Model file for the job. Use its own axes, mm. A direction names the side the tool comes from. Give positions to 0.01 mm unless a question says otherwise; leave off trailing zeros. Write each loop counter-clockwise with the first axis right and the second up, starting at its lowest first coordinate (ties: lowest second). Pieces come first, ordered by that corner, then holes. Notation, with made-up numbers: (17, 76) - (63, 76) arc R11 ccw to (63, 88) - close; hole circle Ø2 at (19.25, 54). An arc over 180 degrees is marked (long way). One line per item, written item: value. Start each with the question number.
(1) Drop flat-ended pins along their axis: P1, Ø2, axis at x = -17, z = -2, coming from the +Y side; P2, Ø2.5, axis at y = 32.5, z = 0, coming from the +X side. Give the stop position or say it passes through.
(2) Probe L1, parallel to Y at x = -18.8, z = 0; L2, parallel to X at y = 51, z = 4.25 (3 decimals); L3, parallel to Z at x = -18.45, y = 32. List the from-to ranges inside material, lowest first.
(3) Cut at D-D, the plane z = -0.25. State how many separate pieces and enclosed holes the cut face has, and give its area (3 significant figures).
(4) Cut at C-C, the plane y = 42.5. List the corners of the cut face in (x, z) (3 decimals).
(5) Cut at B-B, the plane x = -18.55. List the corners of the cut face in (y, z).
(6) Cut at A-A, the plane y = 32.5. List the corners of the cut face in (x, z) (3 decimals), and give its area (3 significant figures).
(7) 3-axis set-ups, long thin cutter, end or side, ignore diameter. For faces 1 (the face through (-17, 36, 0)), 2 (the face through (-19, 40, -5)), 3 (the face through (-17, 44, 0)): which of +Z, -Z, +X, -X, +Y, -Y reach the whole face in a straight line?
(8) Mould opens along Z. For faces 4 (the face through (-19, 40, 5)), 5 (the face through (-14.646, 40.042, 0.089)), 6 (the face through (-19, 27.5, 0)), 7 (the face through (-19, 31, 0)) say: pulls with the +Z half, pulls with the -Z half, needs draft (parallel to the pull), parting line crosses it, or undercut.
from build123d import *

# Parameters (mm, degrees)
SKETCH1_W           = 10
SKETCH1_H           = 25
SKETCH1_R           = 1.5
BOSS_EXTRUDE1_DEPTH = 2
BOSS_EXTRUDE2_START = -56
BOSS_EXTRUDE2_DEPTH = 8
FILLET1_R           = 1


with BuildPart() as part:
    # Sketch1 → Boss-Extrude1 (new body)
    with BuildSketch(Plane(origin=(-20.145, 0, 0), x_dir=(0, 0, -1), z_dir=(1, 0, 0))):
        with Locations((0, 40)):
            Rectangle(SKETCH1_W, SKETCH1_H)
        with Locations((0, 47.5)):
            Circle(SKETCH1_R, mode=Mode.SUBTRACT)
        with Locations((0, 32.5)):
            Circle(SKETCH1_R, mode=Mode.SUBTRACT)
    extrude(amount=BOSS_EXTRUDE1_DEPTH)

    # Sketch2 → Boss-Extrude2 (add)
    with BuildSketch(Plane(origin=(0, 100, 0), x_dir=(1, 0, 0), z_dir=(0, 1, 0)).offset(BOSS_EXTRUDE2_START)):
        with BuildLine():
            Line((-19.645, 5), (-19.645, -5))
            ThreePointArc((-19.645, -5), (-14.645, 0), (-19.645, 5))
        make_face()
    extrude(amount=-BOSS_EXTRUDE2_DEPTH)

    # Fillet1
    fillet1_edges = [part.edges().sort_by_distance(p)[0] for p in [
        (-14.645, 36, 0),
        (-14.645, 44, 0),
    ]]
    fillet(fillet1_edges, radius=FILLET1_R)


solid = part.part
Answers follow:
1. P1: stops at y = 44
1. P2: passes through
2. L1: y = 27.5 to 31, 34 to 46, 49 to 52.5
2. L2: x = -20.145 to -18.145
2. L3: z = -5 to -1.41, 1.41 to 5
3. separate pieces: 3
3. enclosed holes: 0
3. area: 65.7 mm²
4. outline: (-20.145, -5) - (-18.145, -5) - (-18.145, -4.77) arc R5 ccw to (-18.145, 4.77) - (-18.145, 5) - (-20.145, 5) - close
5. outline: (27.5, -5) - (52.5, -5) - (52.5, 5) - (27.5, 5) - close; hole circle Ø3 at (32.5, 0); hole circle Ø3 at (47.5, 0)
6. outline: (-20.145, -5) - (-18.145, -5) - (-18.145, -1.5) - (-20.145, -1.5) - close; (-20.145, 1.5) - (-18.145, 1.5) - (-18.145, 5) - (-20.145, 5) - close
6. area: 14.0 mm²
7. face 1: +Z, -Z, +X, -Y
7. face 2: -Z, +X, -X, +Y, -Y
7. face 3: +Z, -Z, +X, +Y
8. face 4: pulls with the +Z half
8. face 5: parting line crosses it
8. face 6: needs draft
8. face 7: undercut
